The listing builds one solid part. Answer for the finished solid, in the listing's coordinates (mm). Face numbers are marked on the shaded views. Give positions to 0.01 mm unless a question says otherwise; leave off trailing zeros. Order: outer loops, then holes, each group sorted by start corner. A loop starts at its lowest first (then second) coordinate and runs counter-clockwise, first axis right, second up. Notation, with made-up numbers: (54.5, 51.25) - (91.5, 51.25) arc R10 ccw to (91.5, 69.25) - close; hole circle Ø2 at (45, 6). An arc over 180 degrees is marked (long way). Answer in a Markdown table with one row per item. Add a question column.
```python
from build123d import *

# Parameters (mm, degrees)
SKETCH1_R           = 1.27
BOSS_EXTRUDE5_DEPTH = 5.08


with BuildPart() as part:
    # Sketch1 → Boss-Extrude5 (new body)
    with BuildSketch(Plane(origin=(0, 0, 0), x_dir=(1, 0, 0), z_dir=(0, 1, 0))):
        with BuildLine():
            Line((0, 6.405373718), (0, 12.781326863))
            ThreePointArc((0, 12.781326863), (8.247768787, 8.719637674), (11.161688458, 0))
            ThreePointArc((11.161688458, 0), (7.57811845, -7.133507881), (0, -9.643693024))
            ThreePointArc((0, -9.643693024), (-6.018946269, -6.487677618), (-8.043344095, 0))
            ThreePointArc((-8.043344095, 0), (-5.348268381, 4.868517964), (0, 6.405373718))
        make_face()
        Circle(SKETCH1_R, mode=Mode.SUBTRACT)
    extrude(amount=BOSS_EXTRUDE5_DEPTH)


solid = part.part
```
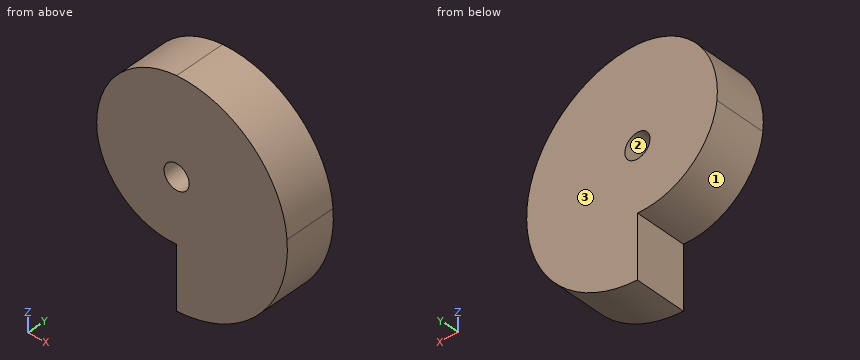
(1) Find section A-A, the plane y = 0.4. Write down the section's boundary in (x, z).
(2) Straight lines are drawn through the part: line 1 (X direction, y = 2.9, z = 0.5); line 2 (Z direction, x = -0.5, y = 2.35); line 3 (X direction, y = 3.2, z = 6.75). For each, find the intervals that lie inside material, in ascending order.
(3) Find section B-B, the plane z = -7.5. Write down the section's boundary in (x, y), plus the area to 3 significant figures.
(4) Each of these flat-tipped pins is pushed along its axis until it touches: P1, Ø3, axis at x = 4, y = 2, coming from the +Z side (3 decimals); P2, Ø4, axis at x = 0, z = 0, coming from the +Y side; P3, Ø2, axis at x = -6, y = 1.5, coming from the +Z side; P4, Ø1.5, axis at x = -2, y = 1, coming from the -Z side. Where does it stop, or does it pass through?
(5) The mould has two halves that part along Z. Classify the marked faces 1, 2 and 3: +Z half, -Z half, draft (parallel to the pull), parting line (faces both ways), or undercut.
(6) Find section C-C, the plane x = 9.25. Write down the section's boundary in (y, z), plus the area to 3 significant figures.
Answer key:
| question | item | result |
|---|---|---|
| 1 | outline | (-8.04, 0) arc R7.27 ccw to (0, -6.41) - (0, -12.78) arc R11.94 ccw to (11.16, 0) arc R10.43 ccw to (0, 9.64) arc R8.88 ccw to start; hole circle Ø2.54 at (0, 0) |
| 2 | line 1 | -8.07 to -1.17, 1.17 to 11.11 |
| 2 | line 2 | -6.44 to -1.17, 1.17 to 9.58 |
| 2 | line 3 | -5.79 to 8 |
| 3 | outline | (0, 0) - (9.18, 0) - (9.18, 5.08) - (0, 5.08) - close |
| 3 | area | 46.6 mm² |
| 4 | P1 | z = 9.525 |
| 4 | P2 | y = 5.08 |
| 4 | P3 | z = 7.52 |
| 4 | P4 | z = -6.44 |
| 5 | face 1 | -Z half |
| 5 | face 2 | undercut |
| 5 | face 3 | draft |
| 6 | outline | (0, -7.4) - (5.08, -7.4) - (5.08, 5.3) - (0, 5.3) - close |
| 6 | area | 64.5 mm² |
